```python
from build123d import *

# Parameters (mm, degrees)
SKETCH1_R           = 1.4
BOSS_EXTRUDE1_DEPTH = 15
SKETCH3_R           = 3
CUT_EXTRUDE2_DEPTH  = 3
SKETCH4_R           = 3
CUT_EXTRUDE3_DEPTH  = 10
BOSS_EXTRUDE2_DEPTH = 5
SKETCH7_R           = 3
CUT_EXTRUDE4_DEPTH  = 5


with BuildPart() as part:
    # Sketch1 → Boss-Extrude1 (new body)
    with BuildSketch(Plane(origin=(0, 0, 0), x_dir=(1, 0, 0), z_dir=(0, 1, 0))):
        with BuildLine():
            Line((-26.264799853, -4.189688425), (-26.264799853, -8.189688425))
            ThreePointArc((-26.264799853, -8.189688425), (-25.386120197, -10.311008768), (-23.264799853, -11.189688425))
            Line((-23.264799853, -11.189688425), (14.289498055, -11.189688425))
            Line((14.289498055, -11.189688425), (56.735200147, -11.189688425))
            ThreePointArc((56.735200147, -11.189688425), (58.85652049, -10.311008768), (59.735200147, -8.189688425))
            Line((59.735200147, -8.189688425), (59.735200147, -4.189688425))
            ThreePointArc((59.735200147, -4.189688425), (58.85652049, -2.068368081), (56.735200147, -1.189688425))
            Line((56.735200147, -1.189688425), (-23.264799853, -1.189688425))
            ThreePointArc((-23.264799853, -1.189688425), (-25.386120197, -2.068368081), (-26.264799853, -4.189688425))
        make_face()
        with Locations((-16.264799853, -6.238015415)):
            Circle(SKETCH1_R, mode=Mode.SUBTRACT)
    extrude(amount=BOSS_EXTRUDE1_DEPTH)

    # Sketch3 → Cut-Extrude2 (cut)
    with BuildSketch(Plane.XZ):
        with Locations((-16.264799853, 6.238015415)):
            Circle(SKETCH3_R)
    extrude(amount=-CUT_EXTRUDE2_DEPTH, mode=Mode.SUBTRACT)

    # Sketch4 → Cut-Extrude3 (cut)
    with BuildSketch(Plane(origin=(0, 15, 0), x_dir=(1, 0, 0), z_dir=(0, 1, 0))):
        with Locations((-16.264799853, -6.238015415)):
            Circle(SKETCH4_R)
    extrude(amount=-CUT_EXTRUDE3_DEPTH, mode=Mode.SUBTRACT)

    # Sketch5 → Boss-Extrude2 (add)
    with BuildSketch(Plane.XZ):
        with BuildLine():
            Line((56.735200147, 11.189688425), (41.735200147, 11.189688425))
            Line((41.735200147, 11.189688425), (41.735200147, 20.523996962))
            ThreePointArc((41.735200147, 20.523996962), (42.613879803, 22.645317306), (44.735200147, 23.523996962))
            Line((44.735200147, 23.523996962), (53.735200147, 23.523996962))
            ThreePointArc((53.735200147, 23.523996962), (55.85652049, 22.645317306), (56.735200147, 20.523996962))
            Line((56.735200147, 20.523996962), (56.735200147, 11.189688425))
        make_face()
    extrude(amount=-BOSS_EXTRUDE2_DEPTH)

    # Sketch7 → Cut-Extrude4 (cut)
    with BuildSketch(Plane(origin=(0, 5, 0), x_dir=(1, 0, 0), z_dir=(0, 1, 0))):
        with Locations((49.235200147, -17.523996962)):
            Circle(SKETCH7_R)
    extrude(amount=-CUT_EXTRUDE4_DEPTH, mode=Mode.SUBTRACT)


solid = part.part
```
CAD build for the part. Positions are in the model's coordinates, mm. A direction names the side the tool comes from. Coordinates: 2 decimals unless noted, no trailing zeros. Order: outer loops, then holes, each group sorted by start corner. A loop starts at its lowest first (then second) coordinate and runs counter-clockwise, first axis right, second up.
(1) Mould opens along X. For faces 4 (the face through (55.8, 2.5, 22.7)), 5 (the face through (-19.262, 10.07, 6.106)), 6 (the face through (16, 15, 6)) say: released by +X, released by -X, zero draft, split by the parting line, or undercut.
Solution:
face 4: released by +X
face 5: undercut
face 6: zero draft
(2) Drill centre lines: L1, parallel to Z at x = 49.5, y = 3.75; L2, parallel to Z at x = 5, y = 3.5; L3, parallel to Y at x = 52.5, z = 17. Where is each one in solid material? Low to high.
Solution:
L1: z = 1.19 to 14.54, 20.51 to 23.52
L2: z = 1.19 to 11.19
L3: y = 0 to 5
(3) Saw through at B-B, the plane x = 47. Write the cut outline in (y, z), and give its area (3 significant figures).
Solution:
outline: (0, 1.19) - (15, 1.19) - (15, 11.19) - (5, 11.19) - (5, 15.52) - (0, 15.52) - close; (0, 19.52) - (5, 19.52) - (5, 23.52) - (0, 23.52) - close
area: 192 mm2
(4) Saw through at C-C, the plane y = 13.5. Write the cut outline in (x, z).
Solution:
outline: (-26.26, 4.19) arc R3 ccw to (-23.26, 1.19) - (56.74, 1.19) arc R3 ccw to (59.74, 4.19) - (59.74, 8.19) arc R3 ccw to (56.74, 11.19) - (-23.26, 11.19) arc R3 ccw to (-26.26, 8.19) - close; hole circle Ø6 at (-16.26, 6.24)
(5) Saw through at D-D, the plane y = 2. Write the cut outline in (x, z), and give its area (3 significant figures).
Solution:
outline: (-26.26, 4.19) arc R3 ccw to (-23.26, 1.19) - (56.74, 1.19) arc R3 ccw to (59.74, 4.19) - (59.74, 8.19) arc R3 ccw to (56.74, 11.19) - (56.74, 20.52) arc R3 ccw to (53.74, 23.52) - (44.74, 23.52) arc R3 ccw to (41.74, 20.52) - (41.74, 11.19) - (-23.26, 11.19) arc R3 ccw to (-26.26, 8.19) - close; hole circle Ø6 at (-16.26, 6.24); hole circle Ø6 at (49.24, 17.52)
area: 977 mm2
(6) Saw through at A-A, the plane z = 19.5. Write the cut outline in (x, y).
Solution:
outline: (41.74, 0) - (46.98, 0) - (46.98, 5) - (41.74, 5) - close; (51.49, 0) - (56.74, 0) - (56.74, 5) - (51.49, 5) - close
(7) Pin check, flat tips, straight feed: pin 1 Ø5.5 at (x, z) = (49.24, 17.52) entering from +Y; pin 2 Ø3.5 at (x, z) = (-16.26, 6.24) entering from -Y; pin 3 Ø1.5 at (y, z) = (2, 14.5) entering from -X; pin 4 Ø5 at (y, z) = (3.5, 9.5) entering from -X. Stop position of each tip, or through.
Solution:
pin 1: passes through
pin 2: stops at y = 3
pin 3: stops at x = 41.74
pin 4: stops at x = -26.26
(8) Which spindle directions (+Z, -Z, +X, -X, +Y, -Y) get a long thin tool onto all of the face, cutting with end or side? Do faces 1 (the face through (41.735, 2, 16)), 2 (the face through (51, 5, 14.7)), 3 (the face through (-18.645, 1.479, 4.413)). Say none if no direction does.
Solution:
face 1: +Z, -X, +Y, -Y
face 2: +Z, +X, -X, +Y
face 3: -Y
